Source: CAD feature listing. Evaluate the final solid. Frame: model axes, mm. A direction names the side the tool comes from. Coordinates: 2 decimals unless noted, no trailing zeros. Write each loop counter-clockwise with the first axis right and the second up, starting at its lowest first coordinate (ties: lowest second). Pieces come first, ordered by that corner, then holes. Notation, with made-up numbers: M 71,40 L 119,40 A13 cw 119,55 Z; hole C 19.25,3.25 d5. An arc over 180 degrees is marked long. One line per item, written item: value. Start each with the question number.
Item 1: Mould query, pull axis Y, two halves, no side actions, for faces 4 (the cylindrical face through (-28.574, 76.755, 19.536)), 5 (the flat face through (0, 85, 51)), 6 (the cylindrical face through (-51.37, 52.94, 67.01)). Classes: released by +Y, released by -Y, zero draft, split by the parting line, or undercut.
Item 2: Pin query (flat end, axial travel): P1, Ø18, axis at y = 79.5, z = 33, coming from the +X side; P2, Ø3, axis at y = 51.5, z = 14.5, coming from the -X side; P3, Ø18, axis at x = -6.5, y = 73.5, coming from the -Z side; P4, Ø2, axis at x = 42.5, z = 44.5, coming from the -Y side. Return the tip coordinate at first contact, or that it passes through.
Item 3: Cut plane A-A, the plane x = 0. Output: boundary loops of the cut face in (y, z), then the cut area to 3 significant figures.
Item 4: Ray query, L1, parallel to Y at x = 0, z = 53.5; L2, parallel to Y at x = 0, z = 21; L3, parallel to Z at x = 47, y = 38. Return the intervals inside material, ascending. Write a range as from..to.
Item 5: Cut plane B-B, the plane y = 0. Output: boundary loops of the cut face in (x, z), then the cut area to 4 significant figures.
Item 6: Cut plane C-C, the plane z = 41.5. Output: boundary loops of the cut face in (x, y), then the cut area to 3 significant figures.
Item 7: Cut plane D-D, the plane x = 18.5. Output: boundary loops of the cut face in (y, z), then the cut area to 3 significant figures.
Item 8: Set-up query: faces 1 (the cylindrical face through (72.28, 17.02, 50.11)), 2 (the flat face through (0, 79, 48.782)), 3 (the cylindrical face through (-15.717, -70.776, 35.777)). Return all of +Z, -Z, +X, -X, +Y, -Y with unobstructed straight access to the full face (end or side cutting, diameter ignored); none if empty.
```python
from build123d import *

# Parameters (mm, degrees)
SZKIC1_R                         = 75
DODANIE_WYCI_GNI_CIE1_DEPTH      = 70
SKORUPA1_T                       = -2.5
SZKIC3_W                         = 13
SZKIC3_H                         = 21
WYTNIJ_WYCI_GNI_CIE1_DEPTH       = 60
SZKIC4_W                         = 9
SZKIC4_H                         = 11
WYTNIJ_WYCI_GNI_CIE2_DEPTH       = 60
DODANIE_WYCI_GNI_CIE2_REACH      = 192.066
DODANIE_WYCI_GNI_CIE2_END_RADIUS = 75
SZKIC7_W                         = 60
SZKIC7_H                         = 35
SZKIC8_W                         = 45.5
SZKIC8_H                         = 26.5
WYTNIJ_WYCI_GNI_CIE4_DEPTH       = 30
ZAOKR_GLENIE1_R                  = 5
WYTNIJ_WYCI_GNI_CIE5_DEPTH       = 14
SZKIC10_R                        = 1.5
WYTNIJ_WYCI_GNI_CIE6_DEPTH       = 10
SZYK_KO_OWY1_COUNT               = 4


with BuildPart() as part:
    # Szkic1 → Dodanie-wyci_gni_cie1 (new body)
    with BuildSketch(Plane.XY):
        Circle(SZKIC1_R)
    extrude(amount=DODANIE_WYCI_GNI_CIE1_DEPTH)

    # Skorupa1
    skorupa1_openings = [part.faces().sort_by_distance(p)[0] for p in [
        (0, 0, 70),
    ]]
    offset(amount=SKORUPA1_T, openings=skorupa1_openings, kind=Kind.INTERSECTION)

    # Szkic3 → Wytnij-wyci_gni_cie1 (cut)
    with BuildSketch(Plane(origin=(0, -75, 0), x_dir=(-1, 0, 0), z_dir=(0, -1, 0))):
        with Locations((0, -35)):
            Rectangle(SZKIC3_W, SZKIC3_H)
    extrude(amount=-WYTNIJ_WYCI_GNI_CIE1_DEPTH, mode=Mode.SUBTRACT)

    # Szkic4 → Wytnij-wyci_gni_cie2 (cut)
    with BuildSketch(Plane(origin=(0, -75, 0), x_dir=(-1, 0, 0), z_dir=(0, -1, 0))):
        with Locations((0, -14)):
            Rectangle(SZKIC4_W, SZKIC4_H)
    extrude(amount=-WYTNIJ_WYCI_GNI_CIE2_DEPTH, mode=Mode.SUBTRACT)

    # Dodanie-wyci_gni_cie2: up to this cylinder (the profile starts outside it)
    dodanie_wyci_gni_cie2_end = Plane(origin=(0, 0, 35.532003), z_dir=(0, 0, -1)) * Cylinder(DODANIE_WYCI_GNI_CIE2_END_RADIUS, 535.132, mode=Mode.PRIVATE)
    # Szkic7 → Dodanie-wyci_gni_cie2 (add, up to the surface)
    with BuildSketch(Plane(origin=(0, 85, 0), x_dir=(-1, 0, 0), z_dir=(0, -1, 0)), mode=Mode.PRIVATE) as dodanie_wyci_gni_cie2_sk1:
        with Locations((0, -35.532003496)):
            Rectangle(SZKIC7_W, SZKIC7_H)
    dodanie_wyci_gni_cie2_tool1 = extrude(dodanie_wyci_gni_cie2_sk1.sketch, amount=DODANIE_WYCI_GNI_CIE2_REACH, mode=Mode.PRIVATE) - dodanie_wyci_gni_cie2_end
    add(dodanie_wyci_gni_cie2_tool1.solids().sort_by_distance((0, 85, 35.532003))[0])

    # Szkic8 → Wytnij-wyci_gni_cie4 (cut)
    with BuildSketch(Plane(origin=(0, 85, 0), x_dir=(1, 0, 0), z_dir=(0, 1, 0))):
        with Locations((0, -35.532003496)):
            Rectangle(SZKIC8_W, SZKIC8_H)
    extrude(amount=-WYTNIJ_WYCI_GNI_CIE4_DEPTH, mode=Mode.SUBTRACT)

    # Zaokr_glenie1
    zaokr_glenie1_edges = [part.edges().sort_by_distance(p)[0] for p in [
        (-30, 76.869317712, 18.032003496),
        (-30, 76.869317712, 53.032003496),
        (30, 76.869317712, 18.032003496),
        (30, 76.869317712, 53.032003496),
    ]]
    fillet(zaokr_glenie1_edges, radius=ZAOKR_GLENIE1_R)

    # Szkic9 → Wytnij-wyci_gni_cie5 (cut)
    with BuildSketch(Plane(origin=(75, 0, 0), x_dir=(0, 0, -1), z_dir=(1, 0, 0))):
        with BuildLine():
            Line((-55, -12.979686846), (-55, 12.020313154))
            ThreePointArc((-55, 12.020313154), (-50, 17.020313154), (-45, 12.020313154))
            Line((-45, 12.020313154), (-45, -12.979686846))
            ThreePointArc((-45, -12.979686846), (-50, -17.979686846), (-55, -12.979686846))
        make_face()
    extrude(amount=-WYTNIJ_WYCI_GNI_CIE5_DEPTH, mode=Mode.SUBTRACT)

    # Szkic10 → Wytnij-wyci_gni_cie6 (cut)
    with BuildSketch(Plane(origin=(53.033008589, 53.033008589, 0), x_dir=(0, 0, -1), z_dir=(0.7071067811865512, 0.7071067811865438, 0))):
        with Locations(Location((-66, 0, 0), (0, 0, 90))):
            Circle(SZKIC10_R)
    wytnij_wyci_gni_cie6 = extrude(amount=-WYTNIJ_WYCI_GNI_CIE6_DEPTH, mode=Mode.SUBTRACT)

    # Szyk ko_owy1: Wytnij-wyci_gni_cie6 ×4 about axis
    szyk_ko_owy1_axis = Axis((0, 0, 70), (0, 0, -1))
    for i in range(1, SZYK_KO_OWY1_COUNT):
        add(wytnij_wyci_gni_cie6.rotate(szyk_ko_owy1_axis, i * 360 / SZYK_KO_OWY1_COUNT), mode=Mode.SUBTRACT)


solid = part.part
```
From the geometry:
1. face 4: zero draft
1. face 5: released by +Y
1. face 6: undercut
2. P1: stops at x = 30
2. P2: stops at x = -55.9
2. P3: stops at z = 0
2. P4: stops at y = -62.47
3. outline: M -75,0 L 75,0 L 75,18.03 L 85,18.03 L 85,22.28 L 72.5,22.28 L 72.5,2.5 L -72.5,2.5 L -72.5,8.5 L -75,8.5 Z; M -75,19.5 L -72.5,19.5 L -72.5,24.5 L -75,24.5 Z; M -75,45.5 L -72.5,45.5 L -72.5,70 L -75,70 Z; M 72.5,48.78 L 85,48.78 L 85,53.03 L 75,53.03 L 75,70 L 72.5,70 Z
3. area: 651 mm²
4. L1: y = -75..-72.5, 72.5..75
4. L2: y = -75..-72.5, 72.5..85
4. L3: z = 0..2.5
5. outline: M -75,0 L 75,0 L 75,45 L 72.5,45 L 72.5,2.5 L -72.5,2.5 L -72.5,70 L -75,70 Z; M 72.5,55 L 75,55 L 75,70 L 72.5,70 Z
5. area: 687.5 mm²
6. outline: M -30,68.74 A75 ccw -6.5,-74.72 L -6.5,-72.21 A72.5 cw -22.75,68.84 L -22.75,85 L -30,85 Z; M 6.5,-74.72 A75 ccw 30,68.74 L 30,85 L 22.75,85 L 22.75,68.84 A72.5 cw 6.5,-72.21 Z
6. area: 1,230 mm²
7. outline: M -72.68,0 L 72.68,0 L 72.68,18.03 L 85,18.03 L 85,22.28 L 70.1,22.28 L 70.1,2.5 L -70.1,2.5 L -70.1,70 L -72.68,70 Z; M 70.1,48.78 L 85,48.78 L 85,53.03 L 72.68,53.03 L 72.68,70 L 70.1,70 Z
7. area: 748 mm²
8. face 1: +X
8. face 2: +Y
8. face 3: +Z
